Geometry check sheet. Reference: drawing and pictorial views, mm from the part's lowest x, y, z. A direction names the side the tool comes from. Round coordinates to 2 decimals unless told otherwise and drop trailing zeros. Loops run counter-clockwise (first coordinate to the right, second up) from the corner with the lowest first, then second, coordinate; pieces in that order, holes last. Notation, with made-up numbers: (50.5, 58.25) -> (85.5, 58.25) arc R16 cw to (85.5, 83.25) -> close; hole circle Ø3 at (-18.5, -32.75). An arc over 180 degrees is marked (long way). Write item = value, one per line.
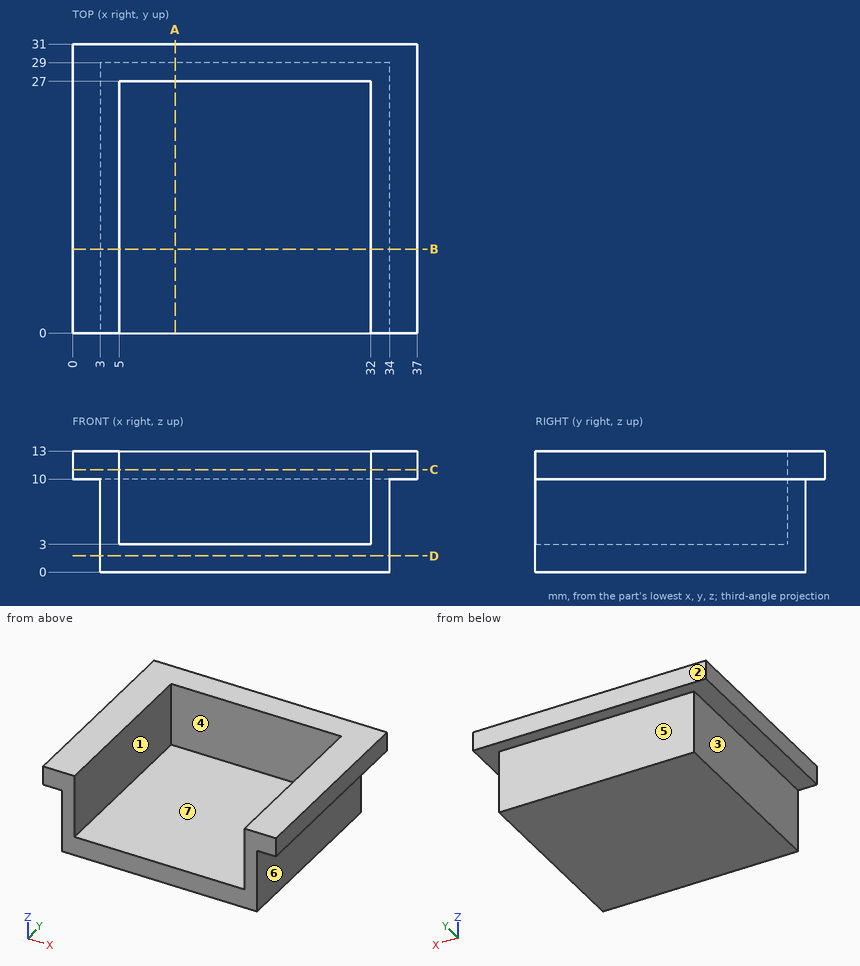
(1) Sectioned sample at D-D, the plane z = 1.75. Record the cut outline in (x, y), and give its area (3 significant figures).
Filled sheet:
outline = (3, 0) -> (34, 0) -> (34, 29) -> (3, 29) -> close
area = 899 mm2
(2) Sectioned sample at A-A, the plane x = 11. Record the cut outline in (y, z).
Filled sheet:
outline = (0, 0) -> (29, 0) -> (29, 10) -> (31, 10) -> (31, 13) -> (27, 13) -> (27, 3) -> (0, 3) -> close
(3) Set-up check for the marked faces 1, 2 and 3: record each of +Z, -Z, +X, -X, +Y, -Y from which the full face is reachable in a straight line by a thin tool's end or side.
Filled sheet:
face_1 = +Z, -Y
face_2 = +Z, -Z, +X, -X, +Y
face_3 = -Z, -X, +Y, -Y
(4) Sectioned sample at C-C, the plane z = 11. Record the cut outline in (x, y).
Filled sheet:
outline = (0, 0) -> (5, 0) -> (5, 27) -> (32, 27) -> (32, 0) -> (37, 0) -> (37, 31) -> (0, 31) -> close
(5) Go/stop test with flat-tipped pins: pin 1 Ø5 at (x, z) = (17, 6) entering from -Y; pin 2 Ø3 at (y, z) = (15.5, 5.5) entering from -X; pin 3 Ø4 at (x, z) = (21.5, 2.5) entering from +Y. Record where each tip stops, or that it passes through.
Filled sheet:
pin_1 = 27
pin_2 = 3
pin_3 = 29
(6) Draft check along X on the marked faces 4, 5, 6 and 7. Enter one of: released by +X, released by -X, zero draft, split by the parting line, or undercut.
Filled sheet:
face_4 = undercut
face_5 = zero draft
face_6 = released by +X
face_7 = undercut
(7) Material ranges on probe 1 along X at (y, z) = (10.5, 9); probe 2 along X at (y, z) = (16.5, 11.75); probe 3 along Y at (x, z) = (7, 8), recorded low to high. Write a range as from..to.
Filled sheet:
probe_1 = 3..5, 32..34
probe_2 = 0..5, 32..37
probe_3 = 27..29
(8) Sectioned sample at B-B, the plane y = 9. Record the cut outline in (x, z).
Filled sheet:
outline = (0, 10) -> (3, 10) -> (3, 0) -> (34, 0) -> (34, 10) -> (37, 10) -> (37, 13) -> (32, 13) -> (32, 3) -> (5, 3) -> (5, 13) -> (0, 13) -> close
